Autodesk Inventor part; units mm, degrees
ref_plane "Start Plane" through (0, 0, -12.7) normal (0, 0, 1) x (1, 0, 0)
ref_plane "End Plane" through (0, 0, 612.7) normal (0, 0, 1) x (1, 0, 0)
ref_plane "Work Plane4" through (12.7, 0, -12.7) normal (0, 0.7071, -0.7071) x (1, 0, 0)
ref_plane "Start Plane" through (0, 0, -12.7) normal (0, 0, 1) x (1, 0, 0)
ref_plane "End Plane" through (0, 0, 612.7) normal (0, 0, 1) x (1, 0, 0)
sketch "Sketch" plane through (0, 0, 0) normal (0, 0, 1) x (1, 0, 0)
  line L0 (25.4, 0) -> (0, 0)
  line L1 (0, 0) -> (0, 25.4)
  line L2 (0, 25.4) -> (1.651, 25.4)
  line L3 (3.175, 23.876) -> (3.175, 6.477)
  line L4 (6.477, 3.175) -> (23.876, 3.175)
  line L5 (25.4, 1.651) -> (25.4, 0)
  line L6 (0, -11.0414) -> (0, 31.5385) construction
  line L7 (-11.0414, 0) -> (31.5385, 0) construction
  arc A0 (3.175, 6.477) -> (6.477, 3.175) centre (6.477, 6.477) ccw
  arc A1 (3.175, 23.876) -> (1.651, 25.4) centre (1.651, 23.876) ccw
  arc A2 (25.4, 1.651) -> (23.876, 3.175) centre (23.876, 1.651) ccw
  line L8 (0, 40.0545) -> (0, -19.5574) construction
  line L9 (-19.5574, 0) -> (40.0545, 0) construction
  point P0 (3.175, 25.4)
  point P1 (3.175, 3.175)
  point P2 (25.4, 3.175)
  dimension "d0" = 25.4
  dimension "d1" = 25.4
  dimension "d2" = 3.175
  dimension "d3" = 3.175
  dimension "d10" = 0
  dimension "d11" = 0
  dimension "d14" = 3.302
  dimension "d15" = 1.524
extrude "Body" add sketch "Sketch" along normal up to surface (625.4 mm away) from surface at -12.7
sketch "Sketch3" plane through (0, 0, 0) normal (0, 0, 1) x (1, 0, 0)
  line L0 (0, 0) -> (10, 0)
ref_plane "Work Plane3" through (0, 0, 0) normal (0, -1, 0) x (1, 0, 0)
ref_plane "Work Plane4" through (12.7, 0, -12.7) normal (0, 0.7071, -0.7071) x (1, 0, 0)
split "Split1" plane through (12.7, 0, -12.7) removes the side toward (0, 0.7071, -0.7071)
ref_plane "Work Plane5" through (12.7, 0, 612.7) normal (0, 0.7071, 0.7071) x (1, 0, 0)
split "Split2" plane through (12.7, 0, 612.7) removes the side toward (0, 0.7071, 0.7071)
sketch "Sketch4" plane through (0, 0, 0) normal (0, -1, 0) x (1, 0, 0)
  line L0 (-2, -12.7) -> (12, -12.7)
  line L1 (-2, 612.7) -> (12, 612.7)
  dimension "d17" = 625.4
equation "\"d0\" = G_H"
equation "\"d1\" = G_H"
equation "\"d2\" = G_T"
equation "\"d3\" = G_T"
equation "\"d14\" = G_IR"
equation "\"d15\" = G_ER"
equation "\"d4\" = G_L"
equation "\"G_H\" = 25.4"
equation "\"G_T\" = 3.175"
equation "\"G_ER\" = 1.524"
equation "\"G_IR\" = 3.302"
equation "\"G_L\" = d17"
equation "\"ex\" = 0"
equation "\"G_OFFSET_START\" = 12.7"
equation "\"G_OFFSET_END\" = 12.7"
equation "\"d12\" = -G_OFFSET_START"
equation "\"d13\" = G_OFFSET_END + B_L"
equation "\"B_L\" = 600"
properties part number "AISC - L 1 x 1 x 1/8 - 24.622" material "Steel, Mild"
Could you check a few things on this model? Use its own coordinates, in mm. A direction names the side the tool comes from. Coordinates: 2 decimals unless noted, no trailing zeros. Write each loop counter-clockwise with the first axis right and the second up, starting at its lowest first coordinate (ties: lowest second). Pieces come first, ordered by that corner, then holes. Notation, with made-up numbers: (87, 75) -> (108, 75) arc R21 ccw to (108, 113) -> close; hole circle Ø5 at (80, 39.25). An arc over 180 degrees is marked (long way). Write item = value, one per line. Start each with the question number.
(1) I need wall thicknesses on line 1 (Y direction, x = 9, z = 530.5) (3 decimals); line 2 (Z direction, x = 2, y = 23.75). Which ranges of each line are inside material? Lowest first, please. Write a range as [from, to].
(2) Will these pins go through, and if not, where does the flat tip stop? pin 1 (6 mm diameter, centred on y = 12.5, z = 237, fed in from +X) (3 decimals); pin 2 (2 mm diameter, centred on x = 21.5, z = 364.5, fed in from +Y) (3 decimals); pin 3 (1 mm diameter, centred on x = 7.5, y = 3, fed in from +Z); pin 4 (4 mm diameter, centred on x = 2.5, z = 95.5, fed in from -Y).
(3) I want a section at A-A (z = 410.5). Please give me the cut outline in (x, y) (3 decimals), plus the area to 3 significant figures.
(4) Which directions (+Z, -Z, +X, -X, +Y, -Y) give clear straight access to the entire face, cutting with the end or side of a thin tool? Please do faces 1 (the face through (0, 13, 296)), 2 (the face through (3.175, 15, 296)).
(5) I want a section at B-B (x = 15). Please give me the cut outline in (y, z) (3 decimals).
Result set:
q1.line_1 = [0, 3.175]
q1.line_2 = [11.05, 588.95]
q2.pin_1 = 3.175
q2.pin_2 = 3.175
q2.pin_3 = 610.2
q2.pin_4 = 0
q3.outline = (0, 0) -> (25.4, 0) -> (25.4, 1.651) arc R1.524 ccw to (23.876, 3.175) -> (6.477, 3.175) arc R3.302 cw to (3.175, 6.477) -> (3.175, 23.876) arc R1.524 ccw to (1.651, 25.4) -> (0, 25.4) -> close
q3.area = 153 mm2
q4.face_1 = +Z, -Z, -X, +Y, -Y
q4.face_2 = +Z, -Z, +X, +Y
q5.outline = (0, -12.7) -> (3.175, -9.525) -> (3.175, 609.525) -> (0, 612.7) -> close
